Part print with two shaded views. Sizes in mm from the minimum x, y, z corner. A direction names the side the tool comes from. Round coordinates to 2 decimals unless told otherwise and drop trailing zeros. Loops run counter-clockwise (first coordinate to the right, second up) from the corner with the lowest first, then second, coordinate; pieces in that order, holes last. Notation, with made-up numbers: (41, -32.75) - (84, -32.75) arc R21 cw to (84, -28.75) - close; hole circle Ø8 at (-4, 45). An arc over 180 degrees is marked (long way). Use a Markdown table: item, result.
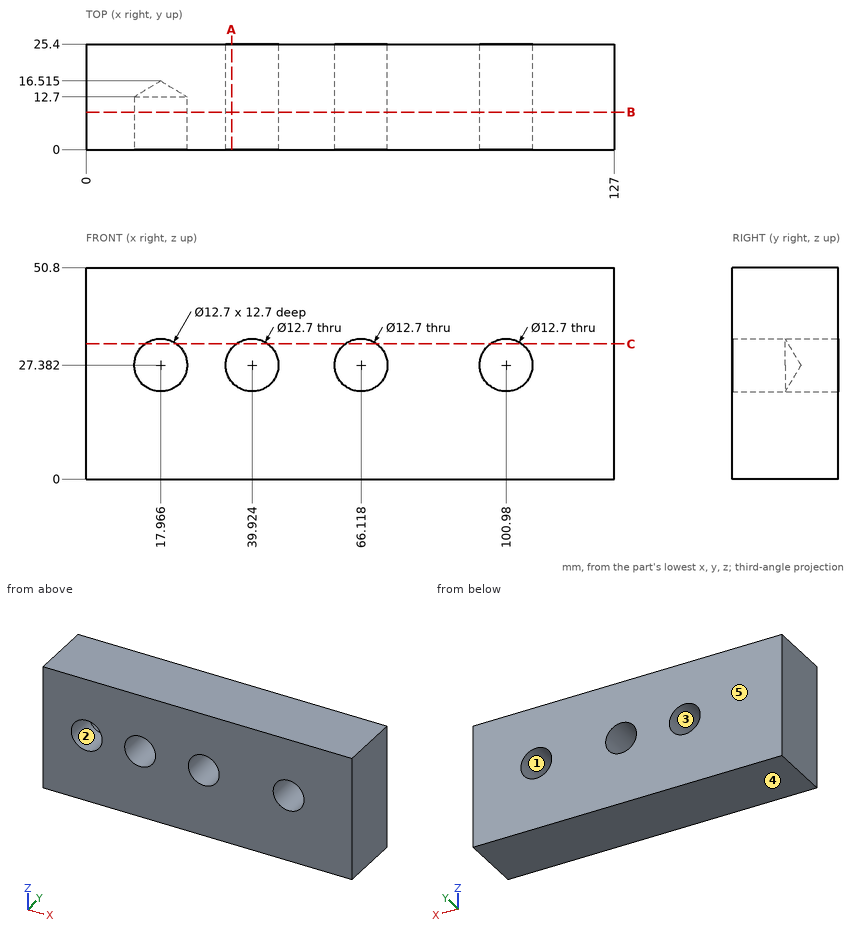
Q1. Cut at A-A, the plane x = 35. List the corners of the cut face in (y, z).
Results found:
| item | result |
|---|---|
| outline | (0, 0) - (25.4, 0) - (25.4, 23.37) - (0, 23.37) - close; (0, 31.39) - (25.4, 31.39) - (25.4, 50.8) - (0, 50.8) - close |
Q2. Drop a flat-ended pin along its axis: pin 1 (11.5 mm diameter, centred on x = 39.92, z = 27.38, fed in from -Y). Give the stop position or say it passes through.
Results found:
| item | result |
|---|---|
| pin 1 | passes through |
Q3. Cut at C-C, the plane z = 32.5. Count the separate pieces of the cut face and the enclosed holes in it, plus the area to 3 significant figures.
Results found:
| item | result |
|---|---|
| separate pieces | 4 |
| enclosed holes | 0 |
| area | 2,550 mm2 |
Q4. Cut at B-B, the plane y = 9. List the corners of the cut face in (x, z).
Results found:
| item | result |
|---|---|
| outline | (0, 0) - (127, 0) - (127, 50.8) - (0, 50.8) - close; hole circle Ø12.7 at (17.97, 27.38); hole circle Ø12.7 at (39.92, 27.38); hole circle Ø12.7 at (66.12, 27.38); hole circle Ø12.7 at (100.98, 27.38) |
Q5. Pull direction Z, two halves, no side cores. Call the marked faces 3, 4 and 5: pulls with the +Z half, pulls with the -Z half, needs draft (parallel to the pull), parting line crosses it, or undercut.
Results found:
| item | result |
|---|---|
| face 3 | undercut |
| face 4 | pulls with the -Z half |
| face 5 | needs draft |
Q6. Which spindle directions (+Z, -Z, +X, -X, +Y, -Y) get a long thin tool onto all of the face, cutting with end or side? Do the marked faces 1 and 2. Say none if no direction does.
Results found:
| item | result |
|---|---|
| face 1 | +Y, -Y |
| face 2 | -Y |
Q7. Probe line 1 (X direction, y = 5.75, z = 28) (1 decimal); line 2 (X direction, y = 8.25, z = 21.5) (1 decimal); line 3 (X direction, y = 16.5, z = 24.5) (1 decimal). List the from-to ranges inside material, lowest first.
Results found:
| item | result |
|---|---|
| line 1 | x = 0 to 11.6, 24.3 to 33.6, 46.2 to 59.8, 72.4 to 94.7, 107.3 to 127 |
| line 2 | x = 0 to 15.6, 20.4 to 37.5, 42.3 to 63.7, 68.5 to 98.6, 103.4 to 127 |
| line 3 | x = 0 to 34.3, 45.6 to 60.5, 71.8 to 95.3, 106.6 to 127 |
